from build123d import *

# Parameters (mm, degrees)
SKETCH1_W                      = 20
SKETCH1_H                      = 37
BOSS_EXTRUDE1_DEPTH            = 12
SKETCH2_W                      = 12
SKETCH2_H                      = 14
CUT_EXTRUDE1_DEPTH             = 14.5
CHAMFER1_SIZE                  = 3
FILLET1_R                      = 3
SKETCH3_W                      = 3
SKETCH3_H                      = 7.7
CUT_EXTRUDE2_DEPTH             = 4.000000008
SKETCH4_W                      = 3
SKETCH4_H                      = 4
CUT_EXTRUDE3_DEPTH             = 4
F_3_3_3_3_DIAMETER_HOLE1_D     = 3.3
F_3_3_3_3_DIAMETER_HOLE1_DEPTH = 8
F_3_3_3_3_DIAMETER_HOLE1_TIP   = 0.991420021


with BuildPart() as part:
    # Sketch1 → Boss-Extrude1 (new body)
    with BuildSketch(Plane(origin=(0, 0, 0), x_dir=(0, 0, -1), z_dir=(1, 0, 0))):
        Rectangle(SKETCH1_W, SKETCH1_H)
    extrude(amount=BOSS_EXTRUDE1_DEPTH)

    # Sketch2 → Cut-Extrude1 (cut)
    with BuildSketch(Plane.XZ.offset(18.5)):
        with Locations((6, 0)):
            Rectangle(SKETCH2_W, SKETCH2_H)
    extrude(amount=-CUT_EXTRUDE1_DEPTH, mode=Mode.SUBTRACT)

    # Chamfer1
    chamfer1_edges = [part.edges().sort_by_distance(p)[0] for p in [
        (0, -18.5, -8.5),
        (0, 18.5, 0),
        (0, -18.5, 8.5),
    ]]
    chamfer(chamfer1_edges, length=CHAMFER1_SIZE)

    # Fillet1
    fillet1_edges = [part.edges().sort_by_distance(p)[0] for p in [
        (6, -4, -7),
        (6, -4, 7),
    ]]
    fillet(fillet1_edges, radius=FILLET1_R)

    # Sketch3 → Cut-Extrude2 (cut)
    with BuildSketch(Plane(origin=(12, 0, 0), x_dir=(0, 0, -1), z_dir=(1, 0, 0))):
        with Locations((-8.5, -14.65)):
            Rectangle(SKETCH3_W, SKETCH3_H)
        with Locations((8.5, -14.65)):
            Rectangle(SKETCH3_W, SKETCH3_H)
    extrude(amount=-CUT_EXTRUDE2_DEPTH, mode=Mode.SUBTRACT)

    # Sketch4 → Cut-Extrude3 (cut)
    with BuildSketch(Plane(origin=(7.999999992, 0, 0), x_dir=(0, 0, -1), z_dir=(1, 0, 0))):
        with Locations((-8.5, -12.8)):
            Rectangle(SKETCH4_W, SKETCH4_H)
        with Locations((8.5, -12.8)):
            Rectangle(SKETCH4_W, SKETCH4_H)
    extrude(amount=-CUT_EXTRUDE3_DEPTH, mode=Mode.SUBTRACT)

    # Ø3.3 (3.3) Diameter Hole1
    with Locations(Plane(origin=(12, 0, 0), x_dir=(0, 0, -1), z_dir=(1, 0, 0))):
        with Locations((0, 1), (0, 13.5)):
            Hole(F_3_3_3_3_DIAMETER_HOLE1_D / 2, depth=F_3_3_3_3_DIAMETER_HOLE1_DEPTH)
            with Locations((0, 0, -(F_3_3_3_3_DIAMETER_HOLE1_DEPTH + F_3_3_3_3_DIAMETER_HOLE1_TIP / 2))):  # 118° drill point
                Cone(0, F_3_3_3_3_DIAMETER_HOLE1_D / 2, F_3_3_3_3_DIAMETER_HOLE1_TIP, mode=Mode.SUBTRACT)


solid = part.part
Check sheet for the modelled part. Datum: model origin and axes. Units: mm. A direction names the side the tool comes from. Round coordinates to 2 decimals unless told otherwise and drop trailing zeros. Loops run counter-clockwise (first coordinate to the right, second up) from the corner with the lowest first, then second, coordinate; pieces in that order, holes last. Notation, with made-up numbers: (84.25, 24) -> (117.25, 24) arc R15 cw to (117.25, 52) -> close; hole circle Ø6 at (-7, -27.5). An arc over 180 degrees is marked (long way). Put each result on its own line as item: value. Start each with the question number.
1. Section check B-B (x = 2.25). Enter the section's corners in (y, z).
2. Draft check along Z on faces 4 (the face through (7.94, 0, -1.31)), 5 (the face through (6, -14.8, -8)), 6 (the face through (6, 0, 10)). Enter one of: +Z half, -Z half, draft (parallel to the pull), parting line (faces both ways), or undercut.
3. Section check D-D (x = 10.25). Enter the section's corners in (y, z).
4. Scan lines: probe 1 along Y at (x, z) = (8, 0); probe 2 along Z at (x, y) = (10.25, 13.5); probe 3 along Z at (x, y) = (5, -16.5). Record each from-to range of solid material in increasing order.
5. Gauge pin test, flat ends, axial feed: pin 1 (3.5 mm diameter, centred on y = -17, z = -8.5, fed in from +X); pin 2 (1.5 mm diameter, centred on y = -13.5, z = 8.5, fed in from +X). Record the tip position at first contact, or that the pin passes through.
6. Section check A-A (x = 4.5). Enter the section's corners in (y, z).
7. Section check C-C (y = -6). Enter the section's corners in (x, z), plus the area to 3 significant figures.
8. Access from +Z, -Z, +X, -X, +Y, -Y to the whole of each face (thin tool, end or side, straight path). Record for faces 1 (the face through (3.18, 13.78, 0.04)), 2 (the face through (8, -10.8, -8)), 3 (the face through (6, -4, 0)).
Findings:
1. outline: (-17.75, -10) -> (17.75, -10) -> (17.75, 10) -> (-17.75, 10) -> (-17.75, 7) -> (-7, 7) arc R3 cw to (-4, 4) -> (-4, -4) arc R3 cw to (-7, -7) -> (-17.75, -7) -> close
2. face 4: undercut
2. face 5: draft
2. face 6: +Z half
3. outline: (-10.8, -10) -> (18.5, -10) -> (18.5, 10) -> (-10.8, 10) -> (-10.8, 7) -> (-7, 7) arc R3 cw to (-4, 4) -> (-4, -4) arc R3 cw to (-7, -7) -> (-10.8, -7) -> close; hole circle Ø3.3 at (1, 0); hole circle Ø3.3 at (13.5, 0)
4. probe 1: y = -4 to -0.65, 2.65 to 11.85, 15.15 to 18.5
4. probe 2: z = -10 to -1.65, 1.65 to 10
4. probe 3: z = -10 to -7, 7 to 10
5. pin 1: stops at x = 8
5. pin 2: stops at x = 4
6. outline: (-18.5, -10) -> (-14.8, -10) -> (-14.8, -7) -> (-18.5, -7) -> close; (-18.5, 7) -> (-14.8, 7) -> (-14.8, 10) -> (-18.5, 10) -> close; (-10.8, -10) -> (18.5, -10) -> (18.5, 10) -> (-10.8, 10) -> (-10.8, 7) -> (-7, 7) arc R3 cw to (-4, 4) -> (-4, -4) arc R3 cw to (-7, -7) -> (-10.8, -7) -> close; hole circle Ø3.3 at (1, 0); hole circle Ø3.3 at (13.5, 0)
7. outline: (0, -10) -> (12, -10) -> (12, -6.83) -> (0, -6.83) -> close; (0, 6.83) -> (12, 6.83) -> (12, 10) -> (0, 10) -> close
7. area: 76.1 mm^2
8. face 1: +X
8. face 2: +Z, -Z, +X
8. face 3: +X, -X, -Y
